Input: dimensioned drawing with shaded views. Units: mm. Origin: part minimum x, y, z. Round coordinates to 2 decimals unless told otherwise and drop trailing zeros. Loops run counter-clockwise (first coordinate to the right, second up) from the corner with the lowest first, then second, coordinate; pieces in that order, holes last.
1) Section A-A, the plane x = 3. Return loops of the section in (y, z).
2) Section B-B, the plane y = 4.2. Return loops of the section in (x, z).
3) Ray query, line 1 along Z through (x, y) = (21, 4.35); line 2 along X through (y, z) = (3.25, 6); line 3 along Z through (x, y) = (2, 5.2). Return the intervals inside material, ascending.
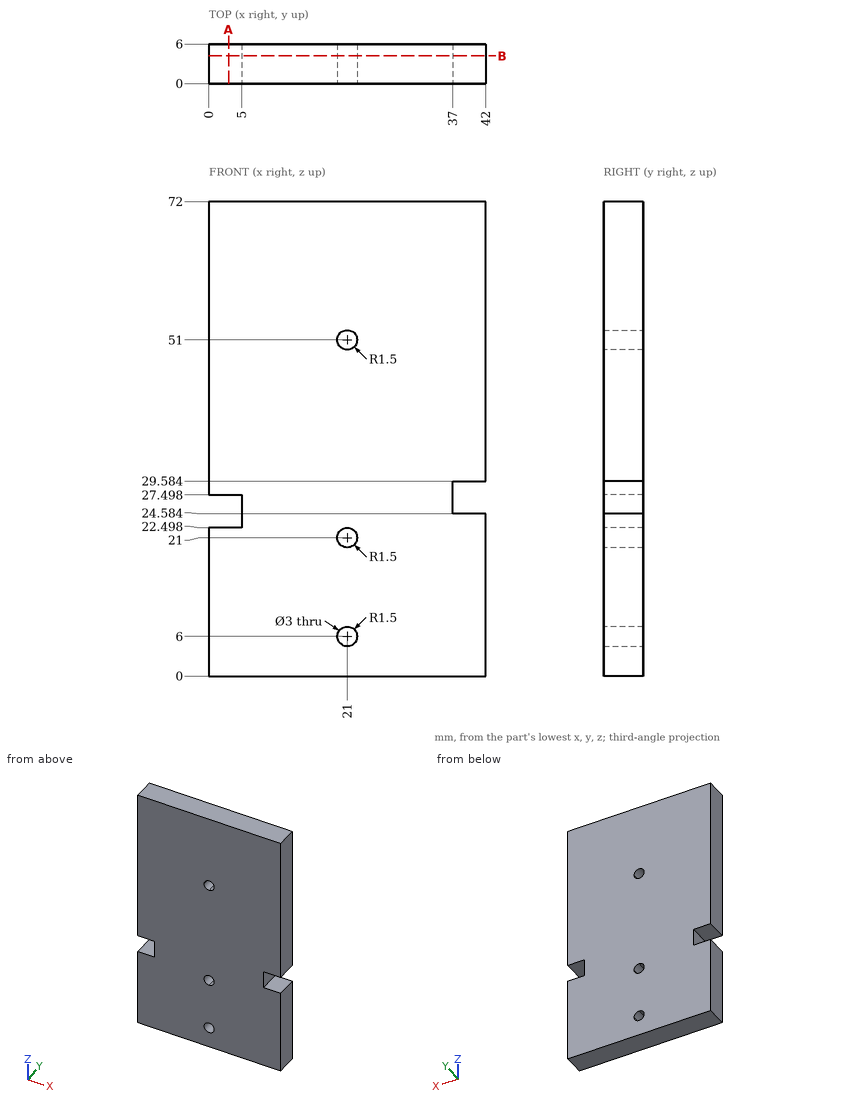
Final values:
1. outline: (0, 0) - (6, 0) - (6, 22.5) - (0, 22.5) - close; (0, 27.5) - (6, 27.5) - (6, 72) - (0, 72) - close
2. outline: (0, 0) - (42, 0) - (42, 24.58) - (37, 24.58) - (37, 29.58) - (42, 29.58) - (42, 72) - (0, 72) - (0, 27.5) - (5, 27.5) - (5, 22.5) - (0, 22.5) - close; hole circle Ø3 at (21, 6); hole circle Ø3 at (21, 21); hole (19.5, 51) arc R1.5 ccw to (21, 49.5) arc R1.5 ccw (long way) to start
3. line 1: z = 0 to 4.5, 7.5 to 19.5, 22.5 to 49.5, 52.5 to 72
3. line 2: x = 0 to 19.5, 22.5 to 42
3. line 3: z = 0 to 22.5, 27.5 to 72
